Verification items for the finished model (mm, model axes). Face numbers are marked on the shaded views. A direction names the side the tool comes from. Coordinates: 2 decimals unless noted, no trailing zeros. Write each loop counter-clockwise with the first axis right and the second up, starting at its lowest first coordinate (ties: lowest second). Pieces come first, ordered by that corner, then holes.
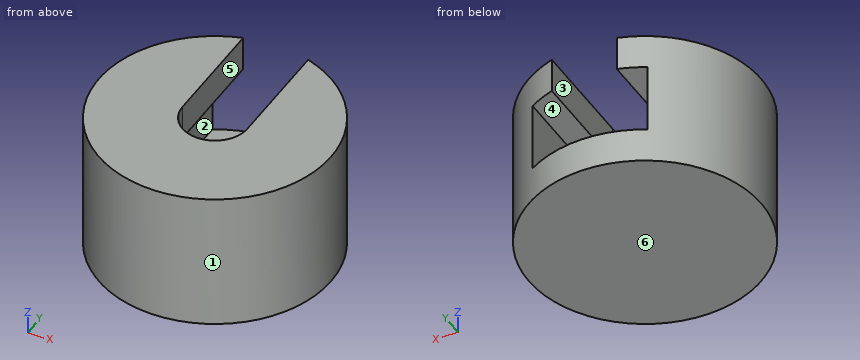
Autodesk Inventor part; units mm, degrees
ref_plane "Work Plane1" through (0, 0, 7.5) normal (0, 0, 1) x (1, 0, 0)
ref_plane "YZ Plane" through (0, 0, 0) normal (1, 0, 0) x (0, 1, 0)
ref_plane "XZ Plane" through (0, 0, 0) normal (0, 1, 0) x (-1, 0, 0)
sketch "Sketch1" plane through (0, 0, 0) normal (0, 0, 1) x (1, 0, 0)
  point P0 (0, 0)
sketch "Sketch2" plane through (0, 0, 0) normal (0, 0, 1) x (1, 0, 0)
  circle A0 centre (0, 0) radius 12.5
  dimension "d0" = 25
extrude "Extrusion1" add sketch "Sketch2" along normal blind 15
ref_plane "Work Plane1" through (0, 0, 7.5) normal (0, 0, 1) x (1, 0, 0)
sketch "Sketch3" plane through (0, 0, 7.5) normal (0, 0, 1) x (1, 0, 0)
  line L0 (6.2, -3.5796) -> (0, -7.1591)
  line L1 (0, -7.1591) -> (-6.2, -3.5796)
  line L2 (-6.2, -3.5796) -> (-6.2, 3.5796)
  line L3 (-6.2, 3.5796) -> (0, 7.1591)
  line L4 (0, 7.1591) -> (6.2, 3.5796)
  line L5 (6.2, 3.5796) -> (6.2, -3.5796)
  point P0 (0, 0)
  point P1 (0, 0)
  dimension "d4" = 12.4
extrude "Extrusion2" cut sketch "Sketch3" along normal mid plane 7.5
sketch "Sketch4" plane through (0, 0, 0) normal (0, 1, 0) x (-1, 0, 0)
  line L0 (6.2, 11.25) -> (0, 11.25)
  line L1 (-6.2, 3.75) -> (0, 3.75)
  line L2 (6.2, 11.25) -> (-6.2, 11.25)
  line L3 (-6.2, 11.25) -> (-6.2, 3.75)
  line L4 (-6.2, 3.75) -> (6.2, 3.75)
  line L5 (6.2, 3.75) -> (6.2, 11.25)
  point P0 (0, 0)
extrude "Extrusion3" cut sketch "Sketch4" along normal blind 15
sketch "Sketch5" plane through (0, 0, 15) normal (0, 0, 1) x (1, 0, 0)
  circle A0 centre (0, 0) radius 12.5
hole "Hole1" at (0, 0, 15) direction (0, 0, -1) diameter 7 depth 7.5
sketch "Sketch6" plane through (0, 0, 15) normal (0, 0, 1) x (1, 0, 0)
  point P0 (0, 0)
sketch "Sketch7" plane through (0, 0, 0) normal (0, 1, 0) x (-1, 0, 0)
  line L0 (3.5, 11.25) -> (-3.5, 11.25)
  line L1 (-3.5, 15) -> (3.5, 15)
  line L2 (3.5, 11.25) -> (-3.5, 11.25)
  line L3 (-3.5, 11.25) -> (-3.5, 15)
  line L4 (-3.5, 15) -> (3.5, 15)
  line L5 (3.5, 15) -> (3.5, 11.25)
  point P0 (0, 0)
extrude "Extrusion4" cut sketch "Sketch7" along normal blind 15
properties part number "Acople tornillo M8"
1. Draft check along Z on the marked faces 4, 5 and 6. Enter one of: pulls with the +Z half, pulls with the -Z half, needs draft (parallel to the pull), parting line crosses it, or undercut.
2. Sectioned sample at C-C, the plane x = -9. Record the boundary of the cut face in (y, z), and give its area (3 significant figures).
3. Sectioned sample at B-B, the plane z = 13. Record the boundary of the cut face in (x, y), and give its area (3 significant figures).
4. Tool access check on the marked faces 1, 2 and 3. Record the directions out of +Z, -Z, +X, -X, +Y, -Y that give a thin tool (end or side, any length) a straight path to the whole face; none if there is none.
5. Gauge pin test, flat ends, axial feed: P1, Ø2, axis at y = 6, z = 7.5, coming from the +X side; P2, Ø3, axis at y = 4.5, z = 13, coming from the +X side; P3, Ø2, axis at y = 7, z = 5, coming from the +X side. Record the tip position at first contact, or that the pin passes through.
6. Material ranges on L1, parallel to Z at x = 3, y = -4.75; L2, parallel to X at y = 0.25, z = 7.5; L3, parallel to Z at x = 0.5, y = 0.75, recorded low to high.
7. Sectioned sample at A-A, the plane y = 4. Record the boundary of the cut face in (x, z), and give its area (3 significant figures).
8. Sectioned sample at D-D, the plane y = 1. Record the boundary of the cut face in (x, z), and give its area (3 significant figures).
Outcome:
1. face 4: undercut
1. face 5: needs draft
1. face 6: pulls with the -Z half
2. outline: (-8.67, 0) - (8.67, 0) - (8.67, 15) - (-8.67, 15) - close
2. area: 260 mm2
3. outline: (-3.5, 0) - (-3.5, 12) arc R12.5 ccw (long way) to (3.5, 12) - (3.5, 0) arc R3.5 cw to start
3. area: 385 mm2
4. face 1: +Z, -Z
4. face 2: +Y
4. face 3: +Z, +Y
5. P1: stops at x = 11.46
5. P2: stops at x = 12.13
5. P3: stops at x = 10.97
6. L1: z = 0 to 3.75, 11.25 to 15
6. L2: x = -12.5 to -6.2, 6.2 to 12.5
6. L3: z = 0 to 3.75
7. outline: (-11.84, 0) - (11.84, 0) - (11.84, 15) - (3.5, 15) - (3.5, 11.25) - (6.2, 11.25) - (6.2, 3.75) - (-6.2, 3.75) - (-6.2, 11.25) - (-3.5, 11.25) - (-3.5, 15) - (-11.84, 15) - close
7. area: 236 mm2
8. outline: (-12.46, 0) - (12.46, 0) - (12.46, 15) - (3.5, 15) - (3.5, 11.25) - (6.2, 11.25) - (6.2, 3.75) - (-6.2, 3.75) - (-6.2, 11.25) - (-3.5, 11.25) - (-3.5, 15) - (-12.46, 15) - close
8. area: 255 mm2
